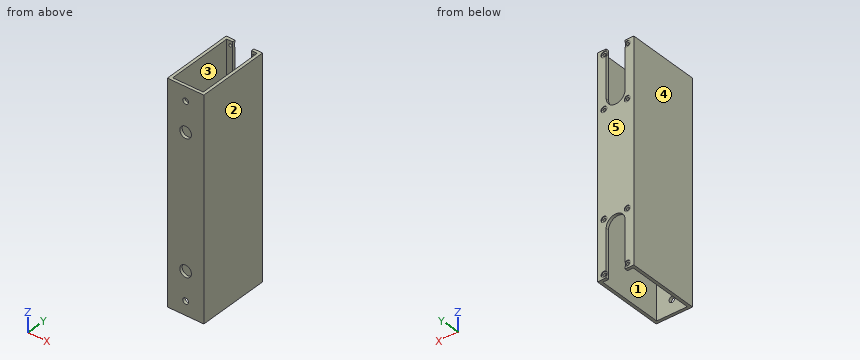
Autodesk Inventor part; units mm, degrees
ref_plane "YZ Plane" through (0, 0, 0) normal (1, 0, 0) x (0, 1, 0)
ref_plane "XZ Plane" through (0, 0, 0) normal (0, 1, 0) x (-1, 0, 0)
ref_plane "XY Plane" through (0, 0, 0) normal (0, 0, 1) x (1, 0, 0)
sketch "スケッチ1" plane through (0, 0, 0) normal (0, 0, 1) x (1, 0, 0)
  line L0 (-12.5, 25) -> (12.5, 25)
  line L1 (12.5, 25) -> (12.5, -25)
  line L2 (12.5, -25) -> (-12.5, -25)
  line L3 (-12.5, -25) -> (-12.5, 25)
  line L4 (-10.5, 23) -> (10.5, 23)
  line L5 (10.5, 23) -> (10.5, -23)
  line L6 (10.5, -23) -> (-10.5, -23)
  line L7 (-10.5, -23) -> (-10.5, 23)
  point P0 (0, 0)
  dimension "d0" = 25
  dimension "d1" = 50
  dimension "d2" = 46
  dimension "d3" = 21
  dimension "d4" = 25
  dimension "d5" = 23
  dimension "d6" = 10.5
  dimension "d7" = 12.5
extrude "押し出し1" add sketch "スケッチ1" along normal blind 150
sketch "スケッチ2" plane through (-12.5, 25, 0) normal (0, 1, 0) x (1, 0, 0)
  line L0 (0, 0) -> (25, 0)
  line L1 (0, 0) -> (0, -150)
  arc A0 (6, -32.5) -> (19, -32.5) centre (12.5, -32.5) ccw
  line L2 (6, -32.5) -> (6, 0)
  line L3 (19, -32.5) -> (19, 0)
  point P0 (12.5, 0)
  dimension "d10" = 13
  dimension "d11" = 32.5
  dimension "d12" = 12.5
extrude "押し出し2" cut sketch "スケッチ2" against normal blind 2
sketch "スケッチ3" plane through (-12.5, 25, 150) normal (0, 1, 0) x (1, 0, 0)
  arc A0 (6, 117.5) -> (19, 117.5) centre (12.5, 117.5) ccw
  circle A1 centre (4.5, 111) radius 1
  circle A2 centre (4.5, 147) radius 1
  circle A3 centre (20.5, 147) radius 1
  circle A4 centre (20.5, 111) radius 1
  point P0 (12.5, 150)
  dimension "d15" = 6.5
  dimension "d16" = 6.5
  dimension "d17" = 2
  dimension "d18" = 8
  dimension "d19" = 8
  dimension "d20" = 8
  dimension "d21" = 8
  dimension "d22" = 29.5
  dimension "d23" = 29.5
hole "穴1" at (-8, 25, 3) at (8, 25, 3) at (8, 25, 39) at (-8, 25, 39) direction (0, -1, 0) diameter 2 depth 2 tip angle 118 counterbore diameter 4 counterbore depth 0.5
sketch "スケッチ4" plane through (-12.5, -25, 0) normal (0, -1, 0) x (1, 0, 0)
  line L0 (25, 0) -> (0, 0)
  line L1 (25, 0) -> (25, 150)
  circle A0 centre (12.5, 9.5) radius 2
  point P0 (12.5, 0)
  dimension "d31" = 4
  dimension "d32" = 12.5
  dimension "d33" = 9.5
hole "穴2" at (0, -25, 9.5) direction (0, 1, 0) diameter 4 end through all
sketch "スケッチ7" plane through (-12.5, -25, 0) normal (0, -1, 0) x (1, 0, 0)
  line L0 (25, 0) -> (25, 150)
  circle A0 centre (12.5, 29) radius 4
  line L1 (25, 0) -> (0, 0)
  point P0 (12.5, 0)
  dimension "d79" = 8
  dimension "d80" = 12.5
  dimension "d88" = 29
hole "穴5" at (0, -25, 29) direction (0, 1, 0) diameter 8 end through all
sketch "スケッチ9" plane through (-12.5, 25, 150) normal (0, 1, 0) x (1, 0, 0)
  line L0 (0, 150) -> (0, 0)
  line L1 (0, 0) -> (25, 0)
  line L2 (6, 0) -> (19, 0)
  line L3 (19, 0) -> (19, 32.5)
  line L4 (6, 32.5) -> (6, 0)
  arc A0 (19, 32.5) -> (6, 32.5) centre (12.5, 32.5) ccw
  point P0 (12.5, 150)
  dimension "d92" = 13
  dimension "d93" = 12.5
  dimension "d95" = 32.5
  dimension "d96" = 6.5
  dimension "d97" = 6.5
extrude "押し出し4" cut sketch "スケッチ9" against normal blind 2
sketch "スケッチ10" plane through (12.5, 25, 150) normal (0, 1, 0) x (1, 0, 0)
  arc A0 (-6, 32.5) -> (-19, 32.5) centre (-12.5, 32.5) ccw
  circle A1 centre (-20.5, 39) radius 1
  circle A2 centre (-20.5, 3) radius 1
  circle A3 centre (-4.5, 3) radius 1
  circle A4 centre (-4.5, 39) radius 1
  point P0 (-12.5, 150)
  dimension "d100" = 2
  dimension "d102" = 16
  dimension "d103" = 16
  dimension "d106" = 8
  dimension "d110" = 8
  dimension "d138" = 6.5
  dimension "d139" = 6.5
  dimension "d140" = 29.5
  dimension "d141" = 29.5
hole "穴6" at (8, 25, 147) at (-8, 25, 147) at (-8, 25, 111) at (8, 25, 111) direction (0, -1, 0) diameter 2 depth 2 tip angle 118 counterbore diameter 4 counterbore depth 0.5
sketch "スケッチ11" plane through (-12.5, -25, 0) normal (0, -1, 0) x (1, 0, 0)
  line L0 (25, 150) -> (0, 150)
  line L1 (25, 0) -> (25, 150)
  circle A0 centre (12.5, 140.5) radius 2
  point P0 (12.5, 0)
  dimension "d118" = 9.5
  dimension "d119" = 4
  dimension "d120" = 12.5
hole "穴7" at (0, -25, 140.5) direction (0, 1, 0) diameter 4 depth 2 tip angle 118
sketch "スケッチ12" plane through (-12.5, -25, 0) normal (0, -1, 0) x (1, 0, 0)
  line L0 (25, 150) -> (0, 150)
  line L1 (25, 0) -> (25, 150)
  circle A0 centre (12.5, 120) radius 4
  point P0 (12.5, 0)
  dimension "d128" = 30
  dimension "d129" = 8
  dimension "d130" = 12.5
hole "穴8" at (0, -25, 120) direction (0, 1, 0) diameter 8 depth 2 tip angle 118
properties part number "07" material "アルミニウム 6061"
Read the model definition and answer for the solid it produces. Units are mm, in the model's axes. Face numbers are marked on the shaded views. A direction names the side the tool comes from. Coordinates: 2 decimals unless noted, no trailing zeros. Loops run counter-clockwise (first coordinate to the right, second up) from the corner with the lowest first, then second, coordinate; pieces in that order, holes last. Notation, with made-up numbers: (2, 58) -> (30, 58) arc R22 cw to (30, 89) -> close; hole circle Ø2 at (-3, 63). An arc over 180 degrees is marked (long way). Answer in a Markdown table with one row per item.
Item 1: A cutting plane is placed at B-B on z = 50.5. Determine the outline of the cut face in (x, y).
Returned:
| item | result |
|---|---|
| outline | (-12.5, -25) -> (12.5, -25) -> (12.5, 25) -> (-12.5, 25) -> close; hole (-10.5, -23) -> (10.5, -23) -> (10.5, 23) -> (-10.5, 23) -> close |
Item 2: For the marked faces 1 and 2, determine the directions among +Z, -Z, +X, -X, +Y, -Y from which every point of the face is accessible in a straight line to the end or side of a thin tool.
Returned:
| item | result |
|---|---|
| face 1 | +Z, -Z |
| face 2 | +Z, -Z, +X, +Y, -Y |
Item 3: A cutting plane is placed at A-A on y = 2. Determine the outline of the cut face in (x, z), plus the area to 3 significant figures.
Returned:
| item | result |
|---|---|
| outline | (-12.5, 0) -> (-10.5, 0) -> (-10.5, 150) -> (-12.5, 150) -> close; (10.5, 0) -> (12.5, 0) -> (12.5, 150) -> (10.5, 150) -> close |
| area | 600 mm^2 |
Item 4: A cutting plane is placed at D-D on z = 120. Determine the outline of the cut face in (x, y).
Returned:
| item | result |
|---|---|
| outline | (-12.5, -25) -> (-4, -25) -> (-4, -23) -> (-10.5, -23) -> (-10.5, 23) -> (-6.5, 23) -> (-6.5, 25) -> (-12.5, 25) -> close; (4, -25) -> (12.5, -25) -> (12.5, 25) -> (6.5, 25) -> (6.5, 23) -> (10.5, 23) -> (10.5, -23) -> (4, -23) -> close |
Item 5: For a pull along X with two mould halves and no side action, classify the marked faces 3, 4 and 5 as released by +X, released by -X, zero draft, split by the parting line, or undercut.
Returned:
| item | result |
|---|---|
| face 3 | undercut |
| face 4 | released by -X |
| face 5 | zero draft |
Item 6: Each of these flat-tipped pins is pushed along its axis until it touches: P1, Ø5, axis at x = 0, z = 29, coming from the -Y side; P2, Ø2.5, axis at x = 8, z = 3, coming from the +Y side; P3, Ø5, axis at x = -8, z = 111, coming from the +Y side; P4, Ø5, axis at x = 0, z = 9.5, coming from the +Y side. Where does it stop, or does it pass through?
Returned:
| item | result |
|---|---|
| P1 | passes through |
| P2 | stops at y = 24.5 |
| P3 | stops at y = 25 |
| P4 | stops at y = -23 |
Item 7: A cutting plane is placed at C-C on z = 9.5. Determine the outline of the cut face in (x, y).
Returned:
| item | result |
|---|---|
| outline | (-12.5, -25) -> (-2, -25) -> (-2, -23) -> (-10.5, -23) -> (-10.5, 23) -> (-6.5, 23) -> (-6.5, 25) -> (-12.5, 25) -> close; (2, -25) -> (12.5, -25) -> (12.5, 25) -> (6.5, 25) -> (6.5, 23) -> (10.5, 23) -> (10.5, -23) -> (2, -23) -> close |
Item 8: Straight lines are drawn through the part: line 1 along Z through (x, y) = (8, 24.75); line 2 along Z through (x, y) = (-8, 24.25); line 3 along X through (y, z) = (-3.5, 115.5). For each, find the intervals that lie inside material, in ascending order. Write a range as [from, to].
Returned:
| item | result |
|---|---|
| line 1 | z = [0, 1], [5, 37], [41, 109], [113, 145], [149, 150] |
| line 2 | z = [0, 2], [4, 38], [40, 110], [112, 146], [148, 150] |
| line 3 | x = [-12.5, -10.5], [10.5, 12.5] |
